Here's how the part is built. I have some questions about the finished solid (model axes, mm). Round coordinates to 2 decimals unless told otherwise and drop trailing zeros. Write each loop counter-clockwise with the first axis right and the second up, starting at its lowest first coordinate (ties: lowest second). Pieces come first, ordered by that corner, then holes. Notation, with made-up numbers: (10, 9) - (56, 9) arc R18 cw to (56, 26) - close; hole circle Ø7 at (77, 79.25). An arc over 180 degrees is marked (long way). One line per item, written item: value. Start each with the question number.
Item 1: Imagine slicing it at D-D, the plane x = -25. Please give me the cut outline in (y, z).
Item 2: Imagine slicing it at A-A, the plane z = 0.5. Please give me the cut outline in (x, y), then the cut area to 3 significant figures.
Item 3: Imagine slicing it at C-C, the plane y = 1.95. Please give me the cut outline in (x, z).
Item 4: For P1, Ø1.5, axis at x = -10, z = -3.5, coming from the -Y side; P2, Ø1.5, axis at y = 2.5, z = -52.5, coming from the +X side, each with a flat end and sliding along its axis, tell me the tip position at first contact or that it passes through.
Item 5: If I drill on line 1 (X direction, y = 1.35, z = 0); line 2 (X direction, y = 1.45, z = -50.5); line 3 (X direction, y = 1.55, z = -41), over which ranges is the centre line in solid material (lowest first)?
Item 6: Imagine slicing it at B-B, the plane x = 0. Please give me the cut outline in (y, z).
Item 7: Thinking about a two-plate mould opening in Z: for faces 1 (the face through (-35, 1, -1)), 2 (the face through (0.631, 1.479, 2.003)), 3 (the face through (-28.346, 1.479, -33.092)), which applies, released by +Z, released by -Z, zero draft, split by the parting line, or undercut?
```python
from build123d import *

# Parameters (mm, degrees)
SKETCH_1_R      = 2.1
EXTRUDE_1_DEPTH = 3
FILLET_1_R      = 3


with BuildPart() as part:
    # 草图1 → 凸台-拉伸1 (new body)
    # profile 1 of 3: a face of its own
    with BuildSketch(Plane(origin=(0, 0, 0), x_dir=(1, 0, 0), z_dir=(0, 1, 0))):
        Polygon((-12.178532268, 10), (8.211170098, 10), (-1.865732489, 60.799005274), (-21.48347839, 56.907470127), align=None)
        with Locations(Location((-4.864418933, 24.522182375, 0), (0, 0, 270))):
            Circle(SKETCH_1_R, mode=Mode.SUBTRACT)
        with Locations(Location((-9.728837866, 49.04436475, 0), (0, 0, 270))):
            Circle(SKETCH_1_R, mode=Mode.SUBTRACT)
    # profile 2 of 3: a face of its own
    with BuildSketch(Plane(origin=(0, 0, 0), x_dir=(1, 0, 0), z_dir=(0, 1, 0))):
        Polygon((12.178532268, -10), (8.211170098, 10), (-12.178532268, 10), (-35, 10), (-35, -10), align=None)
        with Locations(Location((-25, 0, 0), (0, 0, 270))):
            Circle(SKETCH_1_R, mode=Mode.SUBTRACT)
        with Locations(Location((0, 0, 0), (0, 0, 270))):
            Circle(SKETCH_1_R, mode=Mode.SUBTRACT)
    # profile 3 of 3: a face of its own
    with BuildSketch(Plane(origin=(0, 0, 0), x_dir=(1, 0, 0), z_dir=(0, 1, 0))):
        Polygon((-35, 10), (-12.178532268, 10), (-21.48347839, 56.907470127), align=None)
    extrude(amount=EXTRUDE_1_DEPTH)

    # 圆角1
    fillet_1_edges = [part.edges().sort_by_distance(p)[0] for p in [
        (12.178532268, 1.5, 10),
        (-35, 1.5, 10),
        (-35, 1.5, -10),
        (-21.48347839, 1.5, -56.907470127),
        (-1.865732489, 1.5, -60.799005274),
    ]]
    fillet(fillet_1_edges, radius=FILLET_1_R)


solid = part.part
```
Values follow:
1. outline: (0, -44.7) - (3, -44.7) - (3, -2.1) - (0, -2.1) - close; (0, 2.1) - (3, 2.1) - (3, 10) - (0, 10) - close
2. outline: (-35, 0) - (-27.04, 0) - (-27.04, 3) - (-35, 3) - close; (-22.96, 0) - (-2.04, 0) - (-2.04, 3) - (-22.96, 3) - close; (2.04, 0) - (10.29, 0) - (10.29, 3) - (2.04, 3) - close
2. area: 111 mm^2
3. outline: (-35, -9.58) arc R3 ccw to (-34.88, -10.41) - (-21.99, -55.15) arc R3 ccw to (-19.69, -57.26) - (-4.81, -60.22) arc R3 ccw to (-1.28, -57.86) - (11.47, 6.42) arc R3 ccw to (8.52, 10) - (-32, 10) arc R3 ccw to (-35, 7) - close; hole circle Ø4.2 at (-25, 0); hole circle Ø4.2 at (-9.73, -49.04); hole circle Ø4.2 at (-4.86, -24.52); hole circle Ø4.2 at (0, 0)
4. P1: stops at y = 0
4. P2: stops at x = -0.07
5. line 1: x = -35 to -27.1, -22.9 to -2.1, 2.1 to 10.19
5. line 2: x = -23.33 to -11.24, -8.22 to 0.18
5. line 3: x = -26.07 to 2.06
6. outline: (0, -51.39) - (3, -51.39) - (3, -2.1) - (0, -2.1) - close; (0, 2.1) - (3, 2.1) - (3, 10) - (0, 10) - close
7. face 1: zero draft
7. face 2: undercut
7. face 3: released by -Z
